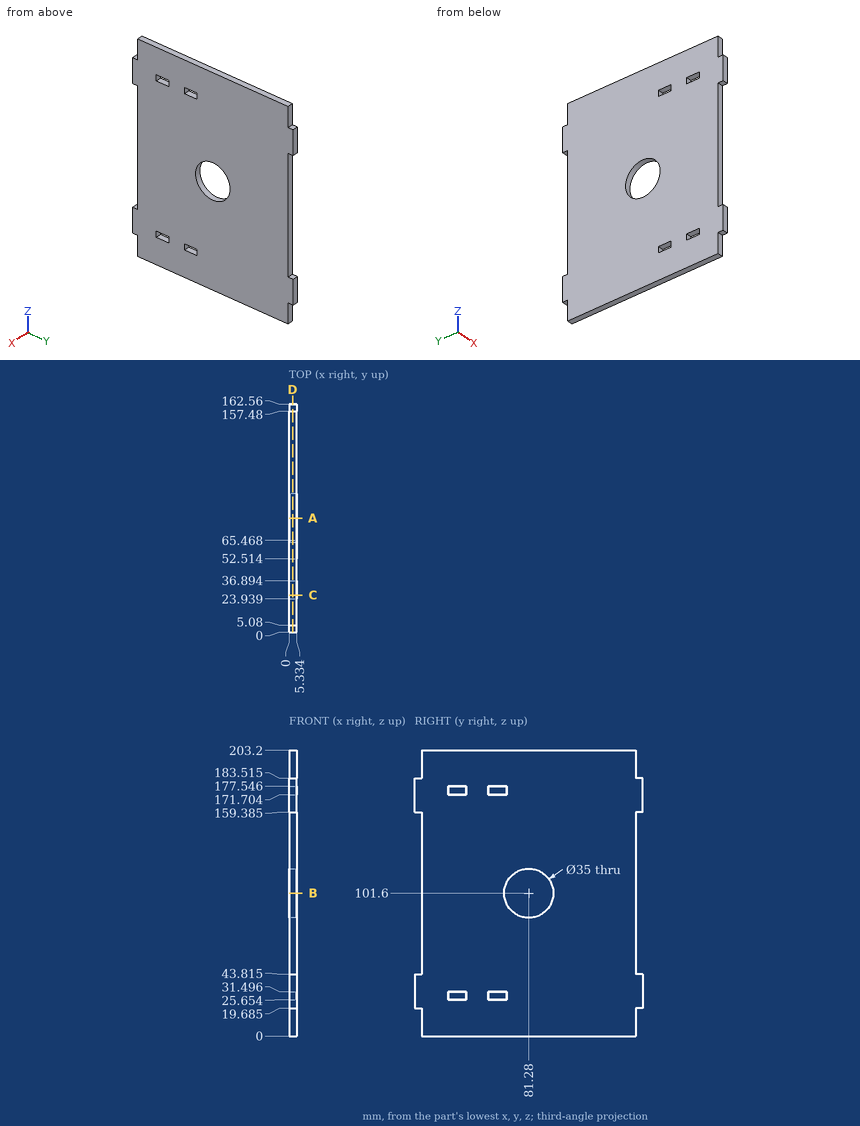
Answer from the drawing. Dimensions are ordinates in mm from the lowest x, y and z of the part. Coordinates: 2 decimals unless noted, no trailing zeros. Write each loop counter-clockwise with the first axis right and the second up, starting at its lowest first coordinate (ties: lowest second). Pieces come first, ordered by that corner, then holes. Notation, with made-up numbers: (-26.75, 34.5) - (-1.75, 34.5) arc R32 ccw to (-1.75, 62.5) - close; hole circle Ø4 at (41, -33.5). An arc over 180 degrees is marked (long way). Return JSON: item names as keys, results as strings.
1. The part is cut by section D-D on x = 2.6. Count the separate pieces of the cut face and the enclosed holes in it, then the cut area to 3 significant figures.
Final values:
{"separate pieces": "1", "enclosed holes": "5", "area": "30,200 mm^2"}
2. This flat-tipped pin is pushed along its axis until it touches: pin 1 Ø2.5 at (x, y) = (3.5, 160) entering from -Z (1 decimal). Where does it stop, or does it pass through?
Final values:
{"pin 1": "z = 19.7"}
3. Consider line 1 along Z through (x, y) = (4, 54.5) (1 decimal); line 2 along Y through (x, z) = (3.8, 101.6); line 3 along Y through (x, z) = (3.05, 46). Determine where each line is inside the solid, lowest interval first.
Final values:
{"line 1": "0 to 25.7, 31.5 to 171.7, 177.5 to 203.2", "line 2": "5.08 to 63.78, 98.78 to 157.48", "line 3": "5.08 to 157.48"}
4. The part is cut by section A-A on y = 81.28. Determine the outline of the cut face in (x, z) (1 decimal).
Final values:
{"outline": "(0, 0) - (5.3, 0) - (5.3, 84.1) - (0, 84.1) - close; (0, 119.1) - (5.3, 119.1) - (5.3, 203.2) - (0, 203.2) - close"}
5. The part is cut by section C-C on y = 26.5. Determine the outline of the cut face in (x, z) (1 decimal), then the cut area to 3 significant figures.
Final values:
{"outline": "(0, 0) - (5.3, 0) - (5.3, 25.7) - (0, 25.7) - close; (0, 31.5) - (5.3, 31.5) - (5.3, 171.7) - (0, 171.7) - close; (0, 177.5) - (5.3, 177.5) - (5.3, 203.2) - (0, 203.2) - close", "area": "1,020 mm^2"}
6. The part is cut by section B-B on z = 101.6. Determine the outline of the cut face in (x, y) (1 decimal), then the cut area to 3 significant figures.
Final values:
{"outline": "(0, 5.1) - (5.3, 5.1) - (5.3, 63.8) - (0, 63.8) - close; (0, 98.8) - (5.3, 98.8) - (5.3, 157.5) - (0, 157.5) - close", "area": "626 mm^2"}
